from build123d import *

# Parameters (mm, degrees)
BOSS_EXTRUDE1_DEPTH   = 20
F_4_CLEARANCE_HOLE1_D = 3.2639
F_6_CLEARANCE_HOLE1_D = 3.7973


with BuildPart() as part:
    # Sketch1 → Boss-Extrude1 (new body)
    with BuildSketch(Plane.XY):
        Polygon((0, 50), (0, 0), (24, 0), (24, 1.5875), (1.5875, 1.5875), (1.5875, 50), align=None)
    boss_extrude1 = extrude(amount=BOSS_EXTRUDE1_DEPTH)

    # #4 Clearance Hole1 (through all)
    with Locations(Plane.ZY):
        with Locations((11.6625, 33.325), (11.6625, 10)):
            f_4_clearance_hole1 = Hole(F_4_CLEARANCE_HOLE1_D / 2)

    # Mirror1: Boss-Extrude1, #4 Clearance Hole1 across plane
    add(boss_extrude1.mirror(Plane(origin=(0, 0, 0), x_dir=(1, 0, 0), z_dir=(0, 0, -1))))
    add(f_4_clearance_hole1.mirror(Plane(origin=(0, 0, 0), x_dir=(1, 0, 0), z_dir=(0, 0, -1))), mode=Mode.SUBTRACT)

    # #6 Clearance Hole1 (through all)
    with Locations(Plane(origin=(0, 0, 0), x_dir=(-1, 0, 0), z_dir=(0, -1, 0))):
        with Locations((-18.2, 0), (-5.8, 0)):
            Hole(F_6_CLEARANCE_HOLE1_D / 2)


solid = part.part
Build history of the part. All positions in model axes, mm. A direction names the side the tool comes from. Give positions to 0.01 mm unless a question says otherwise; leave off trailing zeros. Write each loop counter-clockwise with the first axis right and the second up, starting at its lowest first coordinate (ties: lowest second). Pieces come first, ordered by that corner, then holes. Notation, with made-up numbers: (55.25, -28) - (67.25, -28) arc R24 ccw to (67.25, -12) - close; hole circle Ø1 at (87, 48.5). An arc over 180 degrees is marked (long way). Use one line per item in the form item = value. Start each with the question number.
1. Band-saw the part on B-B on z = 0. Write the cut outline in (x, y), plus the area to 3 significant figures.
2. Band-saw the part on C-C on x = 18.2. Write the cut outline in (y, z), plus the area to 3 significant figures.
3. Band-saw the part on D-D on z = 14. Write the cut outline in (x, y).
4. Drop flat-ended pins along their axis: pin 1 Ø1 at (y, z) = (15, -9.5) entering from +X; pin 2 Ø3.5 at (x, z) = (18.2, 0) entering from +Y; pin 3 Ø12 at (x, y) = (15, 5.5) entering from +Z; pin 4 Ø11 at (x, z) = (9.5, -1) entering from +Y. Give the stop position or say it passes through.
5. Probe line 1 (X direction, y = 40.5, z = -15). List the from-to ranges inside material, lowest first. Write a range as [from, to].
6. 3-axis set-ups, long thin cutter, end or side, ignore diameter. For faces 4 (the face through (13, 1.588, 0)), 5 (the face through (24, 1, 0)): which of +Z, -Z, +X, -X, +Y, -Y reach the whole face in a straight line?
7. Two-plate mould, pull along X, no slides. Class faces 1 (the face through (0, 25, 0)), 2 (the face through (1.588, 25, 0)), 3 (the face through (16.303, 0.805, -0.083)): released by +X, released by -X, zero draft, split by the parting line, or undercut.
8. Band-saw the part on A-A on y = 10. Write the cut outline in (x, z).
Conclusion:
q1.outline = (0, 0) - (3.9, 0) - (3.9, 1.59) - (1.59, 1.59) - (1.59, 50) - (0, 50) - close; (7.7, 0) - (16.3, 0) - (16.3, 1.59) - (7.7, 1.59) - close; (20.1, 0) - (24, 0) - (24, 1.59) - (20.1, 1.59) - close
q1.area = 103 mm²
q2.outline = (0, -20) - (1.59, -20) - (1.59, -1.9) - (0, -1.9) - close; (0, 1.9) - (1.59, 1.9) - (1.59, 20) - (0, 20) - close
q2.area = 57.5 mm²
q3.outline = (0, 0) - (24, 0) - (24, 1.59) - (1.59, 1.59) - (1.59, 50) - (0, 50) - close
q4.pin_1 = 1.59
q4.pin_2 = through
q4.pin_3 = 20
q4.pin_4 = 1.59
q5.line_1 = [0, 1.59]
q6.face_4 = +Z, -Z, +X, +Y
q6.face_5 = +Z, -Z, +X, +Y, -Y
q7.face_1 = released by -X
q7.face_2 = released by +X
q7.face_3 = undercut
q8.outline = (0, -20) - (1.59, -20) - (1.59, -13.29) - (0, -13.29) - close; (0, -10.03) - (1.59, -10.03) - (1.59, 10.03) - (0, 10.03) - close; (0, 13.29) - (1.59, 13.29) - (1.59, 20) - (0, 20) - close
